Here's how the part is built. I have some questions about the finished solid (model axes, mm). Face numbers are marked on the shaded views. A direction names the side the tool comes from. Give positions to 0.01 mm unless a question says otherwise; leave off trailing zeros. Loops run counter-clockwise (first coordinate to the right, second up) from the corner with the lowest first, then second, coordinate; pieces in that order, holes last. Notation, with made-up numbers: (-25.5, -16) - (-15.5, -16) arc R25 ccw to (-15.5, 4) - close; hole circle Ø11 at (0.5, -10). An arc over 180 degrees is marked (long way). Use a Markdown table: item, result.
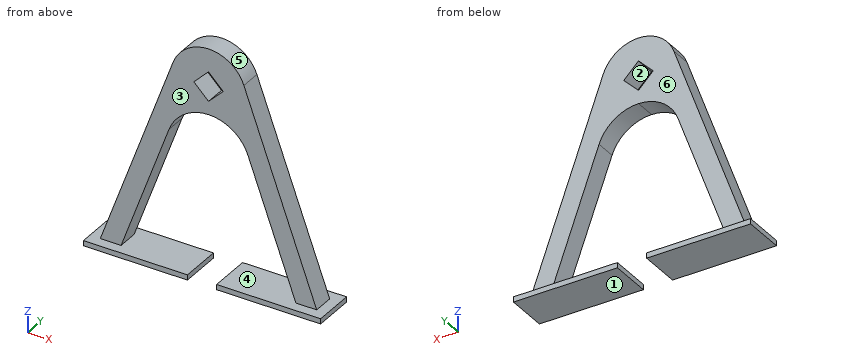
from build123d import *

# Parameters (mm, degrees)
F1_DEPTH = 12.7
F2_W     = 63.5
F2_H     = 25.4
F3_DEPTH = 3.175
F4_W     = 63.5
F4_H     = 25.4
F5_DEPTH = 3.175


with BuildPart() as f1:
    # F0 (on Front) → F1 (new body)
    with BuildSketch(Plane.XZ):
        with BuildLine():
            ThreePointArc((21.59, 7.825371), (0, 22.964419), (-21.59, 7.825371))
            Line((-21.59, 7.825371), (-66.04, -114.3))
            Line((-66.04, -114.3), (-53.34, -114.3))
            Line((-53.34, -114.3), (-24.083093, -33.917308))
            ThreePointArc((-24.083093, -33.917308), (-14.720974, -21.703733), (-0.051192, -17.054196))
            ThreePointArc((-0.051192, -17.054196), (14.679039, -21.674371), (24.083093, -33.917308))
            Line((24.083093, -33.917308), (53.34, -114.3))
            Line((53.34, -114.3), (66.04, -114.3))
            Line((66.04, -114.3), (21.59, 7.825371))
        make_face()
        Polygon((0, 8.980256), (8.980256, 0), (0, -8.980256), (-8.980256, 0), align=None, mode=Mode.SUBTRACT)
    extrude(amount=F1_DEPTH)

    # F2 (on face) → F3 (join)
    with BuildSketch(Plane(origin=(0, 0, -114.3), x_dir=(1, 0, 0), z_dir=(0, 0, -1))):
        with Locations((-40.64, 6.35)):
            Rectangle(F2_W, F2_H)
    extrude(amount=F3_DEPTH)

    # F4 (on face) → F5 (join)
    with BuildSketch(Plane(origin=(0, 0, -114.3), x_dir=(1, 0, 0), z_dir=(0, 0, -1))):
        with Locations((40.64, 6.35)):
            Rectangle(F4_W, F4_H)
    extrude(amount=F5_DEPTH)


solid = f1.part
(1) On a 3-axis mill with a long thin cutter (end or side, diameter ignored), from which of +Z, -Z, +X, -X, +Y, -Y can I reach the whole of each face in a straight line? I mean the marked faces 1, 2 and 3. Say none if no direction works.
A:
| item | result |
|---|---|
| face 1 | -Z, +X, -X, +Y, -Y |
| face 2 | +Y, -Y |
| face 3 | +Z, +X, -X, -Y |
(2) Suppose I cut it at A-A on x = -30. Write out the boundary of the cut face in (y, z) (3 decimals).
A:
| item | result |
|---|---|
| outline | (-19.05, -117.475) - (6.35, -117.475) - (6.35, -114.3) - (-19.05, -114.3) - close; (-12.7, -50.174) - (0, -50.174) - (0, -15.281) - (-12.7, -15.281) - close |
(3) Suppose I cut it at B-B on y = -10. Write out the boundary of the cut face in (x, z) (3 decimals), plus the area to 4 significant figures.
A:
| item | result |
|---|---|
| outline | (-72.39, -117.475) - (-8.89, -117.475) - (-8.89, -114.3) - (-53.34, -114.3) - (-24.083, -33.917) arc R25.629 cw to (-0.051, -17.054) arc R25.629 cw to (24.083, -33.917) - (53.34, -114.3) - (8.89, -114.3) - (8.89, -117.475) - (72.39, -117.475) - (72.39, -114.3) - (66.04, -114.3) - (21.59, 7.825) arc R22.964 ccw to (-21.59, 7.825) - (-66.04, -114.3) - (-72.39, -114.3) - close; hole (-8.98, 0) - (0, -8.98) - (8.98, 0) - (0, 8.98) - close |
| area | 4,605 mm2 |
(4) Suppose I cut it at C-C on z = 6. Write out the boundary of the cut face in (x, y).
A:
| item | result |
|---|---|
| outline | (-22.25, -12.7) - (-2.98, -12.7) - (-2.98, 0) - (-22.25, 0) - close; (2.98, -12.7) - (22.25, -12.7) - (22.25, 0) - (2.98, 0) - close |
(5) Suppose I cut it at D-D on x = 62. Write out the boundary of the cut face in (y, z) (3 decimals).
A:
| item | result |
|---|---|
| outline | (-19.05, -117.475) - (6.35, -117.475) - (6.35, -114.3) - (0, -114.3) - (0, -103.2) - (-12.7, -103.2) - (-12.7, -114.3) - (-19.05, -114.3) - close |
(6) If I drill on line 1 (X direction, y = -2.5, z = -97); line 2 (Z direction, x = -9, y = -14.25) (3 decimals); line 3 (X direction, y = -5, z = -41.5), over which ranges is the centre line in solid material (lowest first)?
A:
| item | result |
|---|---|
| line 1 | -59.74 to -47.04, 47.04 to 59.74 |
| line 2 | -117.475 to -114.3 |
| line 3 | -39.54 to -26.84, 26.84 to 39.54 |
(7) We'd pull the mould along Z, two halves only. Please class the marked faces 4, 5 and 6: pulls with the +Z half, pulls with the -Z half, needs draft (parallel to the pull), parting line crosses it, or undercut.
A:
| item | result |
|---|---|
| face 4 | undercut |
| face 5 | pulls with the +Z half |
| face 6 | needs draft |
(8) Will these pins go through, and if not, where does the flat tip stop? pin 1 (12.5 mm diameter, centred on x = -27.5, y = -2, fed in from +Z); pin 2 (12 mm diameter, centred on y = -5.5, z = -59.5, fed in from +X); pin 3 (1.5 mm diameter, centred on x = 3.5, y = -1, fed in from -Z).
A:
| item | result |
|---|---|
| pin 1 | z = 8.71 |
| pin 2 | x = 48.28 |
| pin 3 | z = -17.41 |
